Could you check a few things on this drawing? It's one solid part, dimensions in mm from its lowest x, y, z. A direction names the side the tool comes from. Round coordinates to 2 decimals unless told otherwise and drop trailing zeros. Order: outer loops, then holes, each group sorted by start corner. A loop starts at its lowest first (then second) coordinate and runs counter-clockwise, first axis right, second up. Notation, with made-up numbers: (38, 25) -> (92, 25) arc R25 cw to (92, 41) -> close; hole circle Ø2 at (69, 73.5). An arc over 180 degrees is marked (long way). Use a Markdown table: item, result. Add a question column.
(1) I want a section at C-C, the plane x = 36. Please give me the cut outline in (y, z) (1 decimal).
(2) I want a section at A-A, the plane y = 76.9. Please give me the cut outline in (x, z), then the cut area to 3 significant figures.
(3) I'm going to push flat-ended pins straight in: P1, Ø3.5, axis at x = 22.5, y = 91.9, coming from the -Z side; P2, Ø10, axis at y = 38, z = 16, coming from the +X side; P3, Ø1, axis at y = 21, z = 17.5, coming from the -X side. Where does each tip first touch, or does it pass through?
(4) If I drill on probe 1 along Y at (x, z) = (22.5, 18.5); probe 2 along X at (y, z) = (69.4, 18.55) (1 decimal); probe 3 along Y at (x, z) = (22.5, 13.5), over which ranges is the centre line in solid material (lowest first)?
(5) Thinking about a two-plate mould opening in Y: for the marked faces 4, 5, 6 and 7, which applies, pulls with the +Y half, pulls with the -Y half, needs draft (parallel to the pull), parting line crosses it, or undercut?
(6) On a 3-axis mill with a long thin cutter (end or side, diameter ignored), from which of +Z, -Z, +X, -X, +Y, -Y can I reach the whole of each face in a straight line? I mean the marked faces 1, 2 and 3. Say none if no direction works.
(7) I want a section at D-D, the plane z = 7. Please give me the cut outline in (x, y) (1 decimal), then the cut area to 3 significant figures.
(8) I want a section at B-B, the plane x = 22.5. Please give me the cut outline in (y, z).
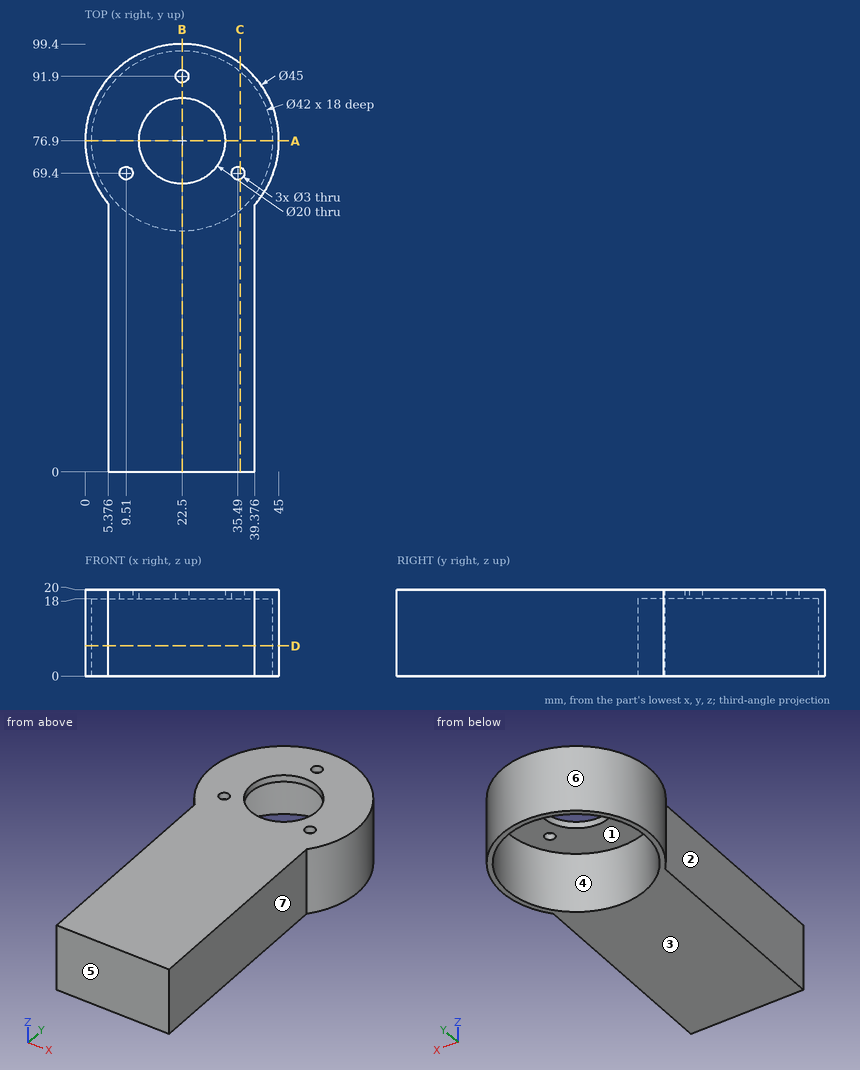
Taken from the geometry:
| question | item | result |
|---|---|---|
| 1 | outline | (0, 0) -> (60.8, 0) -> (60.8, 18) -> (68, 18) -> (68, 20) -> (0, 20) -> close; (70.8, 18) -> (93, 18) -> (93, 0) -> (94.9, 0) -> (94.9, 20) -> (70.8, 20) -> close |
| 2 | outline | (0, 0) -> (1.5, 0) -> (1.5, 18) -> (12.5, 18) -> (12.5, 20) -> (0, 20) -> close; (32.5, 18) -> (43.5, 18) -> (43.5, 0) -> (45, 0) -> (45, 20) -> (32.5, 20) -> close |
| 2 | area | 104 mm2 |
| 3 | P1 | stops at z = 18 |
| 3 | P2 | stops at x = 39.38 |
| 3 | P3 | stops at x = 5.38 |
| 4 | probe 1 | y = 0 to 66.9, 86.9 to 90.4, 93.4 to 99.4 |
| 4 | probe 2 | x = 1.3 to 8, 11 to 15.9, 29.1 to 34, 37 to 43.7 |
| 4 | probe 3 | y = 0 to 55.9, 97.9 to 99.4 |
| 5 | face 4 | undercut |
| 5 | face 5 | pulls with the -Y half |
| 5 | face 6 | parting line crosses it |
| 5 | face 7 | needs draft |
| 6 | face 1 | -Z |
| 6 | face 2 | +Z, -Z, -X, -Y |
| 6 | face 3 | -Z, +X, -X, +Y, -Y |
| 7 | outline | (5.4, 0) -> (39.4, 0) -> (39.4, 62) arc R22.5 ccw (long way) to (5.4, 62.3) -> close; hole circle Ø42 at (22.5, 76.9) |
| 7 | area | 2,140 mm2 |
| 8 | outline | (0, 0) -> (55.9, 0) -> (55.9, 18) -> (66.9, 18) -> (66.9, 20) -> (0, 20) -> close; (86.9, 18) -> (90.4, 18) -> (90.4, 20) -> (86.9, 20) -> close; (93.4, 18) -> (97.9, 18) -> (97.9, 0) -> (99.4, 0) -> (99.4, 20) -> (93.4, 20) -> close |
